```python
from build123d import *
from OCP.BRepFilletAPI import BRepFilletAPI_MakeChamfer

# Parameters (mm, degrees)
SKETCH1_W           = 200
SKETCH1_H           = 100
BOSS_EXTRUDE1_DEPTH = 0.8
SKETCH2_W           = 200
SKETCH2_H           = 100
SKETCH2_W_2         = 198.4
SKETCH2_H_2         = 98.4
BOSS_EXTRUDE2_DEPTH = 15
SKETCH3_W           = 145
SKETCH3_H           = 11.5
BLENDER_DEPTH       = 12
SKETCH3_3_W         = 75
SKETCH3_3_H         = 65
CHARCOALS_DEPTH     = 8
SKETCH3_4_W         = 50
SKETCH3_4_H         = 40
RUBBER_DEPTH        = 10
SKETCH3_5_W         = 21
SKETCH3_5_H         = 40
ERASER_DEPTH        = 12
SKETCH3_6_W         = 35
SKETCH3_6_H         = 35
SHARPENER_DEPTH     = 14.25
CHAMFER1_SIZE       = 10
CHAMFER1_SIZE2      = 5.773502692
SKETCH3_7_W         = 30
SKETCH3_7_H         = 10
CUT_EXTRUDE6_DEPTH  = 9
CHAMFER2_SIZE       = 9.004040443
CHAMFER2_SIZE_2     = 10
SKETCH4_W           = 200
SKETCH4_H           = 100
SKETCH4_W_2         = 198.4
SKETCH4_H_2         = 98.4
BOSS_EXTRUDE3_DEPTH = 7.8
FILLET1_R           = 1
FILLET2_R           = 1.8
FILLET3_R           = 1.8


with BuildPart() as part:
    # Sketch1 → Boss-Extrude1 (new body)
    with BuildSketch(Plane(origin=(0, 0, 0), x_dir=(1, 0, 0), z_dir=(0, 1, 0))):
        Rectangle(SKETCH1_W, SKETCH1_H)
    extrude(amount=-BOSS_EXTRUDE1_DEPTH)

    # Sketch2 → Boss-Extrude2 (add)
    # profile 1 of 2: a face of its own
    with BuildSketch(Plane(origin=(0, 0, 0), x_dir=(1, 0, 0), z_dir=(0, 1, 0))):
        Rectangle(SKETCH2_W, SKETCH2_H)
        Rectangle(SKETCH2_W_2, SKETCH2_H_2, mode=Mode.SUBTRACT)
    # profile 2 of 2: a face of its own
    with BuildSketch(Plane(origin=(0, 0, 0), x_dir=(1, 0, 0), z_dir=(0, 1, 0))):
        Rectangle(SKETCH2_W_2, SKETCH2_H_2)
    extrude(amount=BOSS_EXTRUDE2_DEPTH)

    # Sketch3 → Blender (cut)
    with BuildSketch(Plane(origin=(0, 15, 0), x_dir=(1, 0, 0), z_dir=(0, 1, 0))):
        with Locations((-21.7, -38.45)):
            Rectangle(SKETCH3_W, SKETCH3_H)
    extrude(amount=-BLENDER_DEPTH, mode=Mode.SUBTRACT)

    # Sketch3<3> → Charcoals (cut)
    with BuildSketch(Plane(origin=(0, 15, 0), x_dir=(1, 0, 0), z_dir=(0, 1, 0))):
        with Locations((-56.7, 11.7)):
            Rectangle(SKETCH3_3_W, SKETCH3_3_H)
    extrude(amount=-CHARCOALS_DEPTH, mode=Mode.SUBTRACT)

    # Sketch3<4> → Rubber (cut)
    with BuildSketch(Plane(origin=(0, 15, 0), x_dir=(1, 0, 0), z_dir=(0, 1, 0))):
        with Locations((25.8, 24.2)):
            Rectangle(SKETCH3_4_W, SKETCH3_4_H)
    extrude(amount=-RUBBER_DEPTH, mode=Mode.SUBTRACT)

    # Sketch3<5> → Eraser (cut)
    with BuildSketch(Plane(origin=(0, 15, 0), x_dir=(1, 0, 0), z_dir=(0, 1, 0))):
        with Locations((69.7, 24.2)):
            Rectangle(SKETCH3_5_W, SKETCH3_5_H)
    extrude(amount=-ERASER_DEPTH, mode=Mode.SUBTRACT)

    # Sketch3<6> → Sharpener (cut)
    with BuildSketch(Plane(origin=(0, 15, 0), x_dir=(1, 0, 0), z_dir=(0, 1, 0))):
        with Locations((76.7, -26.7)):
            Rectangle(SKETCH3_6_W, SKETCH3_6_H)
    extrude(amount=-SHARPENER_DEPTH, mode=Mode.SUBTRACT)

    # Chamfer1: one chamfer whose edges measure the first distance from different faces: ONE call of the kernel's chamfer builder (chamfer() names one face for all edges)
    chamfer1_edges_1 = [part.edges().sort_by_distance(p)[0] for p in [
        (-19.2, 15, -11.7),
        (80.2, 15, -24.2),
    ]]
    chamfer1_side_1 = [part.faces().sort_by_distance(p)[0] for p in [
        (11.550891669, 15, 3.081461272),
    ]]
    chamfer1_edges_2 = [part.edges().sort_by_distance(p)[0] for p in [
        (76.7, 15, 9.2),
    ]]
    chamfer1_side_2 = [part.faces().sort_by_distance(p)[0] for p in [
        (76.7, 7.875, 9.2),
    ]]
    chamfer1 = BRepFilletAPI_MakeChamfer(part.part.solid().wrapped)
    for e in chamfer1_edges_1:
        chamfer1.Add(CHAMFER1_SIZE, CHAMFER1_SIZE2, e.wrapped, chamfer1_side_1[0].wrapped)  # the first distance lies on this face
    for e in chamfer1_edges_2:
        chamfer1.Add(CHAMFER1_SIZE, CHAMFER1_SIZE2, e.wrapped, chamfer1_side_2[0].wrapped)  # the first distance lies on this face
    add(Compound.cast(chamfer1.Shape()), mode=Mode.REPLACE)

    # Sketch3<7> → Cut-Extrude6 (cut)
    with BuildSketch(Plane(origin=(0, 15, 0), x_dir=(1, 0, 0), z_dir=(0, 1, 0))):
        with Locations((15.8, -27.7)):
            Rectangle(SKETCH3_7_W, SKETCH3_7_H)
    extrude(amount=-CUT_EXTRUDE6_DEPTH, mode=Mode.SUBTRACT)

    # Chamfer2
    # the kernel refuses this chamfer: 10, 9.004040443 mm, written as the material it adds along each edge
    with BuildSketch(Plane(origin=(56.551839571, 6, 22.7), x_dir=(0, 0.9994864482690294, -0.032044340008195435), z_dir=(-1, 0, 0))) as chamfer2_piece_1_section:
        Polygon((CHAMFER2_SIZE * 0.999486448267, -CHAMFER2_SIZE * 0.0320443400081), (-CHAMFER2_SIZE_2 * 0.0320443400082, -CHAMFER2_SIZE_2 * 0.999486448269), (0, 0), align=None)
    chamfer2_piece_1 = extrude(amount=81.503679141, mode=Mode.PRIVATE)
    chamfer2_piece_1 = split(chamfer2_piece_1, bisect_by=Plane(origin=(15.8, 15, 26.033334004), z_dir=(0, -1, 0)), keep=Keep.TOP, mode=Mode.PRIVATE)
    add(chamfer2_piece_1)

    # Sketch4 → Boss-Extrude3 (add)
    with BuildSketch(Plane(origin=(0, 15, 0), x_dir=(1, 0, 0), z_dir=(0, 1, 0))):
        Rectangle(SKETCH4_W, SKETCH4_H)
        Rectangle(SKETCH4_W_2, SKETCH4_H_2, mode=Mode.SUBTRACT)
    extrude(amount=BOSS_EXTRUDE3_DEPTH)

    # Fillet1
    fillet1_edges = [part.edges().sort_by_distance(p)[0] for p in [
        (-99.2, 18.9, -49.2),
        (-99.2, 18.9, 49.2),
        (99.2, 18.9, 49.2),
        (99.2, 18.9, -49.2),
    ]]
    fillet(fillet1_edges, radius=FILLET1_R)

    # Fillet2
    fillet2_edges = [part.edges().sort_by_distance(p)[0] for p in [
        (-100, 11, -50),
        (100, 11, -50),
        (100, 11, 50),
        (-100, 11, 50),
    ]]
    fillet(fillet2_edges, radius=FILLET2_R)

    # Fillet3
    # the kernel refuses this fillet: 1.8 mm, written as the material it adds along each edge
    with BuildSketch(Plane(origin=(50.8, 15, 44.2), x_dir=(0, 0, -1), z_dir=(0, -1, 0)), Plane(origin=(50.8, 15, 32.7), x_dir=(-1, 0, 0), z_dir=(0, -1, 0)), Plane(origin=(59.2, 15, -4.2), x_dir=(1, 0, 0), z_dir=(0, -1, 0))) as fillet3_piece_1:
        with BuildLine():
            CenterArc((FILLET3_R, -FILLET3_R), FILLET3_R, 90, 90)
            Line((0, -FILLET3_R), (0, 0))
            Line((0, 0), (FILLET3_R, 0))
        make_face()
    extrude(amount=12)
    with BuildSketch(Plane(origin=(-94.2, 15, 44.2), x_dir=(0, 0, -1), z_dir=(0, -1, 0)), Plane(origin=(-94.2, 15, 32.7), x_dir=(1, 0, 0), z_dir=(0, -1, 0)), Plane(origin=(59.2, 15, -44.2), x_dir=(1, 0, 0), z_dir=(0, -1, 0))) as fillet3_piece_2:
        with BuildLine():
            CenterArc((FILLET3_R, FILLET3_R), FILLET3_R, 180, 90)
            Line((0, FILLET3_R), (0, 0))
            Line((0, 0), (FILLET3_R, 0))
        make_face()
    extrude(amount=12)
    with BuildSketch(Plane(origin=(-19.2, 13.726497308, 20.8), x_dir=(-1, 0, 0), z_dir=(0, -1, 0))) as fillet3_piece_3_section:
        with BuildLine():
            CenterArc((FILLET3_R, FILLET3_R), FILLET3_R, 180, 90)
            Line((0, FILLET3_R), (0, 0))
            Line((0, 0), (FILLET3_R, 0))
        make_face()
    fillet3_piece_3 = extrude(amount=11.226497308, mode=Mode.PRIVATE)
    fillet3_piece_3 = split(fillet3_piece_3, bisect_by=Plane(origin=(-20.005000388, 8.761730117, 20.378537809), z_dir=(0.5000000000000009, -0.8660254037844382, 0)), keep=Keep.TOP, mode=Mode.PRIVATE)
    add(fillet3_piece_3)
    with BuildSketch(Plane(origin=(-94.2, 15, 20.8), x_dir=(1, 0, 0), z_dir=(0, -1, 0)), Plane(origin=(-94.2, 15, -44.2), x_dir=(0, 0, 1), z_dir=(0, -1, 0))) as fillet3_piece_4:
        with BuildLine():
            CenterArc((FILLET3_R, -FILLET3_R), FILLET3_R, 90, 90)
            Line((0, -FILLET3_R), (0, 0))
            Line((0, 0), (FILLET3_R, 0))
        make_face()
    extrude(amount=12.5)
    with BuildSketch(Plane(origin=(-19.2, 13.726497308, -44.2), x_dir=(-1, 0, 0), z_dir=(0, -1, 0))) as fillet3_piece_5_section:
        with BuildLine():
            CenterArc((FILLET3_R, -FILLET3_R), FILLET3_R, 90, 90)
            Line((0, -FILLET3_R), (0, 0))
            Line((0, 0), (FILLET3_R, 0))
        make_face()
    fillet3_piece_5 = extrude(amount=11.226497308, mode=Mode.PRIVATE)
    fillet3_piece_5 = split(fillet3_piece_5, bisect_by=Plane(origin=(-20.005000388, 8.761730117, -43.778537809), z_dir=(0.5000000000000009, -0.8660254037844382, 0)), keep=Keep.TOP, mode=Mode.PRIVATE)
    add(fillet3_piece_5)
    with BuildSketch(Plane(origin=(50.8, 15, -4.2), x_dir=(-1, 0, 0), z_dir=(0, -1, 0)), Plane(origin=(50.8, 15, -44.2), x_dir=(0, 0, 1), z_dir=(0, -1, 0))) as fillet3_piece_6:
        with BuildLine():
            CenterArc((FILLET3_R, FILLET3_R), FILLET3_R, 180, 90)
            Line((0, FILLET3_R), (0, 0))
            Line((0, 0), (FILLET3_R, 0))
        make_face()
    extrude(amount=14.5)
    with BuildSketch(Plane(origin=(0.8, 15, -4.2), x_dir=(1, 0, 0), z_dir=(0, -1, 0)), Plane(origin=(0.8, 15, -44.2), x_dir=(0, 0, 1), z_dir=(0, -1, 0))) as fillet3_piece_7:
        with BuildLine():
            CenterArc((FILLET3_R, -FILLET3_R), FILLET3_R, 90, 90)
            Line((0, -FILLET3_R), (0, 0))
            Line((0, 0), (FILLET3_R, 0))
        make_face()
    extrude(amount=14.5)
    with BuildSketch(Plane(origin=(80.2, 13.726497308, -4.2), x_dir=(-1, 0, 0), z_dir=(0, -1, 0))) as fillet3_piece_8_section:
        with BuildLine():
            CenterArc((FILLET3_R, FILLET3_R), FILLET3_R, 180, 90)
            Line((0, FILLET3_R), (0, 0))
            Line((0, 0), (FILLET3_R, 0))
        make_face()
    fillet3_piece_8 = extrude(amount=10.726497308, mode=Mode.PRIVATE)
    fillet3_piece_8 = split(fillet3_piece_8, bisect_by=Plane(origin=(78.509719514, 8.250613415, -4.608516769), z_dir=(0.5000000000000009, -0.8660254037844382, 0)), keep=Keep.TOP, mode=Mode.PRIVATE)
    add(fillet3_piece_8)
    with BuildSketch(Plane(origin=(80.2, 13.726497308, -44.2), x_dir=(-1, 0, 0), z_dir=(0, -1, 0))) as fillet3_piece_9_section:
        with BuildLine():
            CenterArc((FILLET3_R, -FILLET3_R), FILLET3_R, 90, 90)
            Line((0, -FILLET3_R), (0, 0))
            Line((0, 0), (FILLET3_R, 0))
        make_face()
    fillet3_piece_9 = extrude(amount=10.726497308, mode=Mode.PRIVATE)
    fillet3_piece_9 = split(fillet3_piece_9, bisect_by=Plane(origin=(78.509719514, 8.250613415, -43.791483231), z_dir=(0.5000000000000009, -0.8660254037844382, 0)), keep=Keep.TOP, mode=Mode.PRIVATE)
    add(fillet3_piece_9)
    with BuildSketch(Plane(origin=(94.2, 9.5, 9.2), x_dir=(0, 0, 1), z_dir=(0, -1, 0))) as fillet3_piece_10_section:
        with BuildLine():
            CenterArc((FILLET3_R, FILLET3_R), FILLET3_R, 180, 90)
            Line((0, FILLET3_R), (0, 0))
            Line((0, 0), (FILLET3_R, 0))
        make_face()
    fillet3_piece_10 = extrude(amount=8.75, mode=Mode.PRIVATE)
    fillet3_piece_10 = split(fillet3_piece_10, bisect_by=Plane(origin=(93.765274696, 3.031109619, 10.336739391), z_dir=(0, -0.500000000000001, -0.866025403784438)), keep=Keep.TOP, mode=Mode.PRIVATE)
    add(fillet3_piece_10)
    with BuildSketch(Plane(origin=(94.2, 15, 44.2), x_dir=(-1, 0, 0), z_dir=(0, -1, 0)), Plane(origin=(59.2, 15, 44.2), x_dir=(0, 0, -1), z_dir=(0, -1, 0))) as fillet3_piece_11:
        with BuildLine():
            CenterArc((FILLET3_R, FILLET3_R), FILLET3_R, 180, 90)
            Line((0, FILLET3_R), (0, 0))
            Line((0, 0), (FILLET3_R, 0))
        make_face()
    extrude(amount=14.25)
    with BuildSketch(Plane(origin=(59.2, 9.5, 9.2), x_dir=(0, 0, 1), z_dir=(0, -1, 0))) as fillet3_piece_12_section:
        with BuildLine():
            CenterArc((FILLET3_R, -FILLET3_R), FILLET3_R, 90, 90)
            Line((0, -FILLET3_R), (0, 0))
            Line((0, 0), (FILLET3_R, 0))
        make_face()
    fillet3_piece_12 = extrude(amount=8.75, mode=Mode.PRIVATE)
    fillet3_piece_12 = split(fillet3_piece_12, bisect_by=Plane(origin=(59.634725304, 3.031109619, 10.336739391), z_dir=(0, -0.500000000000001, -0.866025403784438)), keep=Keep.TOP, mode=Mode.PRIVATE)
    add(fillet3_piece_12)
    # the kernel refuses this fillet: 1.8 mm, written as the material it takes off along each edge
    with BuildSketch(Plane(origin=(0.8, 19.5, 32.7), x_dir=(0, 0, -1), z_dir=(0, -1, 0))) as fillet3_2_piece_1_section:
        with BuildLine():
            CenterArc((FILLET3_R, -FILLET3_R), FILLET3_R, 90, 90)
            Line((0, -FILLET3_R), (0, 0))
            Line((0, 0), (FILLET3_R, 0))
        make_face()
    fillet3_2_piece_1 = extrude(amount=18, mode=Mode.PRIVATE)
    fillet3_2_piece_1 = split(fillet3_2_piece_1, bisect_by=Plane(origin=(0.390952326, 8.287487107, 30.159488191), z_dir=(0, 0.7431448254771393, 0.6691306063591413)), keep=Keep.TOP, mode=Mode.PRIVATE)
    add(fillet3_2_piece_1, mode=Mode.SUBTRACT)
    with BuildSketch(Plane(origin=(30.8, 19.5, 32.7), x_dir=(1, 0, 0), z_dir=(0, -1, 0))) as fillet3_2_piece_2_section:
        with BuildLine():
            CenterArc((FILLET3_R, -FILLET3_R), FILLET3_R, 90, 90)
            Line((0, -FILLET3_R), (0, 0))
            Line((0, 0), (FILLET3_R, 0))
        make_face()
    fillet3_2_piece_2 = extrude(amount=18, mode=Mode.PRIVATE)
    fillet3_2_piece_2 = split(fillet3_2_piece_2, bisect_by=Plane(origin=(31.209047674, 8.287487107, 30.159488191), z_dir=(0, 0.7431448254771393, 0.6691306063591413)), keep=Keep.TOP, mode=Mode.PRIVATE)
    add(fillet3_2_piece_2, mode=Mode.SUBTRACT)


solid = part.part
```
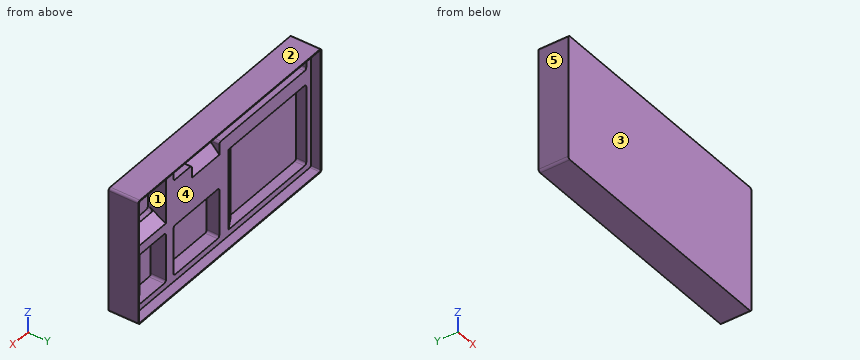
Could you check a few things on this model? Use its own coordinates, in mm. Face numbers are marked on the shaded views. A direction names the side the tool comes from. Give positions to 0.01 mm unless a question says otherwise; leave off trailing zeros. Write each loop counter-clockwise with the first axis right and the second up, starting at its lowest first coordinate (ties: lowest second). Pieces come first, ordered by that corner, then holes. Notation, with made-up numbers: (-13.75, 15.5) - (20.25, 15.5) arc R25 cw to (20.25, 40.5) - close; hole circle Ø3 at (11.25, 13). An arc over 180 degrees is marked (long way). One line per item, written item: value. Start each with the question number.
Item 1: I'm going to push flat-ended pins straight in: pin 1 (10.5 mm diameter, centred on x = 70, z = 30.5, fed in from +Y); pin 2 (4 mm diameter, centred on x = -50, z = -16, fed in from +Y); pin 3 (23 mm diameter, centred on x = 66, z = -18.5, fed in from +Y). Where does each tip first touch, or does it pass through?
Item 2: Which directions (+Z, -Z, +X, -X, +Y, -Y) give clear straight access to the entire face, cutting with the end or side of a thin tool? Please do the marked faces 4 and 5.
Item 3: Please list where these lines run through material, in increasing order: line 1 (Z direction, x = 38.5, y = 12); line 2 (X direction, y = 7.5, z = -17); line 3 (Z direction, x = 82, y = 18.5). Write a range as from..to.
Item 4: If we mould it in two halves opening along Z, with no side actions, what happens to the marked faces 1, 2 and 3? For each: +Z half, -Z half, draft (parallel to the pull), parting line (faces both ways), or undercut.
Item 5: Imagine slicing it at A-A, the plane z = 39. List the corners of the cut face in (x, y) for me, and give its area (3 significant figures).
Item 6: Imagine slicing it at C-C, the plane z = -21.5. List the corners of the cut face in (x, y) for me.
Item 7: Imagine slicing it at D-D, the plane x = -39.5. List the corners of the cut face in (y, z) for me.
Item 8: Imagine slicing it at B-B, the plane x = 54. List the corners of the cut face in (y, z) for me, and give its area (3 significant figures).
Geometry says:
1. pin 1: y = 0.75
1. pin 2: y = 7
1. pin 3: y = 15
2. face 4: +Y
2. face 5: +Z, -Z, -X, +Y, -Y
3. line 1: -50..-44.2, -4.2..32.7, 44.2..50
3. line 2: -100..-94.2, -19.2..0.8, 50.8..59.2, 80.2..100
3. line 3: -50..-49.2, 49.2..50
4. face 1: undercut
4. face 2: +Z half
4. face 3: draft
5. outline: (-100, -0.8) - (100, -0.8) - (100, 22.8) - (99.2, 22.8) - (99.2, 15) - (94.2, 15) - (94.2, 0.75) - (59.2, 0.75) - (59.2, 15) - (50.8, 15) - (50.8, 3) - (-94.2, 3) - (-94.2, 15) - (-99.2, 15) - (-99.2, 22.8) - (-100, 22.8) - close
5. area: 934 mm^2
6. outline: (-100, -0.8) - (100, -0.8) - (100, 22.8) - (99.2, 22.8) - (99.2, 15) - (90.2, 15) - (80.2, 9.23) - (80.2, 3) - (59.2, 3) - (59.2, 15) - (50.8, 15) - (50.8, 5) - (0.8, 5) - (0.8, 15) - (-9.2, 15) - (-19.2, 9.23) - (-19.2, 7) - (-94.2, 7) - (-94.2, 15) - (-99.2, 15) - (-99.2, 22.8) - (-100, 22.8) - close
7. outline: (-0.8, -50) - (22.8, -50) - (22.8, -49.2) - (15, -49.2) - (15, -44.2) - (7, -44.2) - (7, 20.8) - (15, 20.8) - (15, 32.7) - (3, 32.7) - (3, 44.2) - (15, 44.2) - (15, 49.2) - (22.8, 49.2) - (22.8, 50) - (-0.8, 50) - close
8. outline: (-0.8, -50) - (22.8, -50) - (22.8, -49.2) - (15, -49.2) - (15, 49.2) - (22.8, 49.2) - (22.8, 50) - (-0.8, 50) - close
8. area: 1,590 mm^2
